Autodesk Inventor part; units mm, degrees
ref_plane "YZ Plane" through (0, 0, 0) normal (1, 0, 0) x (0, 1, 0)
ref_plane "XZ Plane" through (0, 0, 0) normal (0, 1, 0) x (-1, 0, 0)
ref_plane "XY Plane" through (0, 0, 0) normal (0, 0, 1) x (1, 0, 0)
sketch "Sketch1" plane through (0, 0, 0) normal (0, 0, 1) x (1, 0, 0)
  circle A0 centre (0, 0) radius 5
  circle A1 centre (0, 0) radius 11
  line L0 (-11, 0) -> (-11, -25)
  line L1 (11, 0) -> (11, -25)
  line L2 (0, 0) -> (0, -54.7816)
  line L3 (-11, -25) -> (-5, -25)
  line L4 (-5, -25) -> (-5, -10)
  line L5 (5, -10) -> (5, -25)
  line L6 (5, -25) -> (11, -25)
  line L7 (-5, -10) -> (5, -10)
  dimension "d0" = 10
  dimension "d1" = 22
  dimension "d4" = 10
  dimension "d6" = 15
  dimension "d22" = 6
  dimension "d23" = 6
extrude "Extrusion1" add sketch "Sketch1" along normal blind 23 contours A0 | A1 L7 | L1 L6 L5 L7 A1 | A1 L7 L4 L3 L0
sketch "Sketch2" plane through (11, -25, 0) normal (1, 0, 0) x (0, 0, -1)
  circle A0 centre (-4, 4) radius 2.1
  line L0 (0, 0) -> (0, 25)
  line L1 (0, 25) -> (-23, 25)
  line L2 (-23, 0) -> (-23, 25)
  line L3 (0, 0) -> (-23, 0)
  dimension "d9" = 4.2
  dimension "d10" = 4
  dimension "d20" = 4
extrude "Extrusion2" cut sketch "Sketch2" against normal through all contours A0
fillet "Fillet1" radius 2 2 edges at (-5, -10, 11.5) (5, -10, 11.5)
sketch "Sketch5" plane through (11, -25, 0) normal (1, 0, 0) x (0, 0, -1)
  circle A0 centre (-4, 4) radius 2.1
  line L0 (0, 0) -> (0, 25)
  line L1 (0, 25) -> (-23, 25)
  line L2 (-23, 0) -> (-23, 25)
  line L3 (0, 0) -> (-23, 0)
  line L4 (-23, 15) -> (0, 15)
  line L5 (0, 15) -> (-23, 15)
  line L6 (-15, 8) -> (0, 8)
  line L7 (0, 8) -> (0, 53.1691)
  line L8 (0, 53.1691) -> (-15, 53.1691)
  line L9 (-15, 53.1691) -> (-15, 8)
  line L10 (0, 0) -> (0, 25)
  line L11 (0, 25) -> (0, 25)
  line L12 (0, 25) -> (-23, 25)
  line L13 (-23, 25) -> (-23, 25)
  line L14 (0, 25) -> (-23, 25)
  dimension "d28" = 4
  dimension "d29" = 15
extrude "Extrusion5" cut sketch "Sketch5" against normal through all contours L6 L9 L4 L0 | L4 L9 L1 L0 | L1 L9 L8 L7
fillet "Fillet2" radius 4 4 edges at (8, -25, 0) (8, -17, 0) (-8, -17, 0) (-8, -25, 0)
fillet "Fillet3" radius 2 2 edges at (8, -17, 15) (-8, -17, 15)
sketch "Sketch6" plane through (0, 0, 23) normal (0, 0, 1) x (1, 0, 0)
  circle A0 centre (0, 0) radius 4.7625
  dimension "d34" = 9.525
extrude "Extrusion6" cut sketch "Sketch6" against normal up to next
properties part number "Piston_Holder" material "Acetal Resin, Black"
Read the model definition and answer for the solid it produces. Units are mm, in the model's axes. A direction names the side the tool comes from. Round coordinates to 2 decimals unless told otherwise and drop trailing zeros. Write each loop counter-clockwise with the first axis right and the second up, starting at its lowest first coordinate (ties: lowest second). Pieces come first, ordered by that corner, then holes. Notation, with made-up numbers: M 33,53.5 L 42,53.5 A20 ccw 42,65.5 Z; hole C -4.5,-5 d1. An arc over 180 degrees is marked long. Use a Markdown table: item, result.
1) For a pull along Y with two mould halves and no side action, classify faces 1 (the cylindrical face through (-8.04, -16.43, 14.4)), 2 (the flat face through (11, -15, 16)), 3 (the cylindrical face through (-7.958, -18.918, 4.273)) as pulls with the +Y half, pulls with the -Y half, needs draft (parallel to the pull), parting line crosses it, or undercut.
Answers follow:
| item | result |
|---|---|
| face 1 | pulls with the +Y half |
| face 2 | needs draft |
| face 3 | undercut |
2) The part is cut by section B-B (x = 0). Write down the section's boundary in (y, z).
Answers follow:
| item | result |
|---|---|
| outline | M -10,15 L -4.76,15 L -4.76,23 L -10,23 Z; M 4.76,15 L 11,15 L 11,23 L 4.76,23 Z |
3) A tool of negligible diameter and unlimited length cuts with its end or side. For faces 4 (the flat face through (0, -10, 19)), 5 (the flat face through (-8, -17, 9)), 6 (the flat face through (-8, -25, 13)), from which of +Z, -Z, +X, -X, +Y, -Y can it reach the whole face along a straight path? Write none if from no direction.
Answers follow:
| item | result |
|---|---|
| face 4 | +Z, -Z, -Y |
| face 5 | -Z, +X, -X, +Y |
| face 6 | +Z, -Z, +X, -X, -Y |
4) Straight lines are drawn through the part: line 1 along Y through (x, z) = (-9.45, 4); line 2 along Y through (x, z) = (0, 21); line 3 along Z through (x, y) = (7.25, -6). For each, find the intervals that lie inside material, in ascending order. Write a range as [from, to].
Answers follow:
| item | result |
|---|---|
| line 1 | y = [-25, -23.1], [-18.9, -17] |
| line 2 | y = [-10, -4.76], [4.76, 11] |
| line 3 | z = [15, 23] |
5) The part is cut by section A-A (z = 11.25). Write down the section's boundary in (x, y).
Answers follow:
| item | result |
|---|---|
| outline | M -11,-25 L -5,-25 L -5,-17 L -11,-17 Z; M 5,-25 L 11,-25 L 11,-17 L 5,-17 Z |
6) The part is cut by section C-C (z = 21.25). Write down the section's boundary in (x, y) (1 decimal).
Answers follow:
| item | result |
|---|---|
| outline | M -11,-25 L -5,-25 L -5,-12 A2 cw -3,-10 L 3,-10 A2 cw 5,-12 L 5,-25 L 11,-25 L 11,0 A11 ccw -11,0 Z; hole C 0,0 d9.5 |
7) Flat-ended cylindrical pins translate along their axes: pin 1 (3 mm diameter, centred on x = 8.5, z = 8, fed in from +Y); pin 2 (4 mm diameter, centred on x = -2.5, z = 18, fed in from -Y); pin 3 (3 mm diameter, centred on x = 7, y = 7, fed in from -Z). Find the tip coordinate at first contact, or state that the pin passes through.
Answers follow:
| item | result |
|---|---|
| pin 1 | stops at y = -17 |
| pin 2 | stops at y = -10.68 |
| pin 3 | stops at z = 15 |
8) The part is cut by section D-D (y = -22). Write down the section's boundary in (x, z), plus the area to 3 significant figures.
Answers follow:
| item | result |
|---|---|
| outline | M -11,0.13 L -5,0.13 L -5,2.15 L -11,2.15 Z; M -11,5.85 L -5,5.85 L -5,23 L -11,23 Z; M 5,0.13 L 11,0.13 L 11,2.15 L 5,2.15 Z; M 5,5.85 L 11,5.85 L 11,23 L 5,23 Z |
| area | 230 mm2 |
